from build123d import *

# Parameters (mm, degrees)
F0_R     = 11
F1_DEPTH = 4
F2_COUNT = 4


with BuildPart() as f1:
    # F0 (on Top) → F1 (new body, symmetric)
    with BuildSketch(Plane.XY):
        with BuildLine():
            ThreePointArc((-17.7828708233, 34.5995821148), (-23.3825877712, 16.6188629138), (-13.9969587461, 0.291797633))
            ThreePointArc((-13.9969587461, 0.291797633), (0, -14), (13.9969587461, 0.291797633))
            ThreePointArc((13.9969587461, 0.291797633), (23.3825877712, 16.6188629138), (17.7828708233, 34.5995821148))
            Line((17.7828708233, 34.5995821148), (8.8914354117, 50))
            Line((8.8914354117, 50), (-8.8914354117, 50))
            Line((-8.8914354117, 50), (-17.7828708233, 34.5995821148))
        make_face()
        Circle(F0_R, mode=Mode.SUBTRACT)
        with BuildLine():
            Line((8.8914354117, 19.1991642296), (16.1812389964, 31.8254744156))
            ThreePointArc((16.1812389964, 31.8254744156), (20.4311974682, 17.2440748743), (13.4930582959, 3.7332797675))
            ThreePointArc((13.4930582959, 3.7332797675), (0, 14), (-13.4930582959, 3.7332797675))
            ThreePointArc((-13.4930582959, 3.7332797675), (-20.4311974682, 17.2440748743), (-16.1812389964, 31.8254744156))
            Line((-16.1812389964, 31.8254744156), (-8.8914354117, 19.1991642296))
            Line((-8.8914354117, 19.1991642296), (8.8914354117, 19.1991642296))
        make_face(mode=Mode.SUBTRACT)
        Polygon((10.2282444271, 40.3837430948), (13.567731326, 34.5995821148), (6.783865663, 22.8495821148), (-6.783865663, 22.8495821148), (-13.567731326, 34.5995821148), (-10.2282444271, 40.3837430948), (-6.783865663, 46.3495821148), (6.783865663, 46.3495821148), align=None, mode=Mode.SUBTRACT)
    extrude(amount=F1_DEPTH, both=True)

    # F2: F1 ×4 about axis
    f2_axis = Axis((0, 0, 4), (0, 0, 1))


with BuildPart() as f1_1:
    add(f1.part)
    for i in range(1, F2_COUNT):
        add(f1.part.rotate(f2_axis, i * 360 / F2_COUNT))


solid = f1_1.part
Here's how the part is built. I have some questions about the finished solid (model axes, mm). A direction names the side the tool comes from. Give positions to 0.01 mm unless a question says otherwise; leave off trailing zeros. Loops run counter-clockwise (first coordinate to the right, second up) from the corner with the lowest first, then second, coordinate; pieces in that order, holes last. Notation, with made-up numbers: (33, 62.5) -> (42, 62.5) arc R23 ccw to (42, 81.5) -> close; hole circle Ø5 at (-0.5, 80.25). An arc over 180 degrees is marked (long way). Answer as a JSON object with one key per item and string values. Group by question number.
Item 1: Imagine slicing it at A-A on y = 29. Write out the boundary of the cut face in (x, z), then the cut area to 3 significant figures.
Item 2: Will these pins go through, and if not, where does the flat tip stop? pin 1 (6 mm diameter, centred on x = -23.5, y = -24.5, fed in from +Z); pin 2 (1.5 mm diameter, centred on y = -10.5, z = 1, fed in from -X); pin 3 (1 mm diameter, centred on y = 33, z = -2.5, fed in from -X); pin 4 (2 mm diameter, centred on x = -27, z = 2.5, fed in from +Y).
Item 3: On a 3-axis mill with a long thin cutter (end or side, diameter ignored), from which of +Z, -Z, +X, -X, +Y, -Y can I reach the whole of each face in a straight line? I mean faces 1 (the flat face through (46.35, 0, 0)), 2 (the flat face through (42.19, -13.4, 0.06)). Say none if no direction works.
Item 4: Imagine slicing it at C-C on z = -1.75. Give the number of separate pieces and of enclosed holes in the cut face, then the cut area to 3 significant figures.
Item 5: Thinking about a two-plate mould opening in X: for faces 3 (the cylindrical face through (21.302, 29.18, 0.056)), 4 (the flat face through (-42.19, 13.4, 0.06)), 5 (the cylindrical face through (10, 9.8, -0.1)), 6 (the cylindrical face through (11.416, -18.991, 0.056)), which applies, pulls with the +X half, pulls with the -X half, needs draft (parallel to the pull), parting line crosses it, or undercut?
Item 6: I need wall thicknesses on L1, parallel to X at y = 0, z = 1; L2, parallel to Y at x = 26, z = -1.75. Which ranges of each line are inside material? Lowest first, please.
Item 7: Imagine slicing it at B-B on x = 26. Write out the boundary of the cut face in (y, z).
Answer list:
{
 "1": {"outline": "(-21.39, -4) -> (-18.03, -4) -> (-18.03, 4) -> (-21.39, 4) -> close; (-14.55, -4) -> (-10.33, -4) -> (-10.33, 4) -> (-14.55, 4) -> close; (10.33, -4) -> (14.55, -4) -> (14.55, 4) -> (10.33, 4) -> close; (18.03, -4) -> (21.39, -4) -> (21.39, 4) -> (18.03, 4) -> close", "area": "121 mm2"},
 "2": {"pin 1": "stops at z = 4", "pin 2": "stops at x = -48.51", "pin 3": "stops at x = -19.4", "pin 4": "stops at y = 22.52"},
 "3": {"face 1": "+Z, -Z", "face 2": "+Z, -Z, +X, -Y"},
 "4": {"separate pieces": "1", "enclosed holes": "21", "area": "2,370 mm2"},
 "5": {"face 3": "pulls with the +X half", "face 4": "pulls with the -X half", "face 5": "undercut", "face 6": "undercut"},
 "6": {"L1": "x = -50 to -46.35, -22.85 to -19.2, -14 to -11, 11 to 14, 19.2 to 22.85, 46.35 to 50", "L2": "y = -22.52 to -19.37, -12.82 to -8.6, 8.6 to 12.82, 19.37 to 22.52"},
 "7": {"outline": "(-22.52, -4) -> (-19.37, -4) -> (-19.37, 4) -> (-22.52, 4) -> close; (-12.82, -4) -> (-8.6, -4) -> (-8.6, 4) -> (-12.82, 4) -> close; (8.6, -4) -> (12.82, -4) -> (12.82, 4) -> (8.6, 4) -> close; (19.37, -4) -> (22.52, -4) -> (22.52, 4) -> (19.37, 4) -> close"}
}
